Geometry: see drawing. Coordinates: mm, zero at the bounding-box minimum. A direction names the side the tool comes from. Give positions to 0.01 mm unless a question says otherwise; leave off trailing zeros. Order: outer loops, then holes, each group sorted by start corner. A loop starts at its lowest first (then second) coordinate and runs counter-clockwise, first axis right, second up. Notation, with made-up numbers: M -10.5,-2.75 L 39.5,-2.75 A17 cw 39.5,15.25 Z; hole C 32,14 d9. An arc over 180 degrees is marked long. Answer as a JSON object with one key per item and string values. Group by question number.
1. Material intervals for L1, parallel to X at y = 19, z = 31; L2, parallel to X at y = 49, z = 17; L3, parallel to Y at x = 16.25, z = 36, sorted ascending. Write a range as [from, to].
2. Section query B-B (x = 10). Output: boundary loops of the cut face in (y, z), plus the area to 3 significant figures.
3. Section query C-C (z = 25). Output: boundary loops of the cut face in (x, y), plus the area to 3 significant figures.
4. Section query D-D (y = 38). Output: boundary loops of the cut face in (x, z), plus the area to 3 significant figures.
5. Pin query (flat end, axial travel): P1, Ø4, axis at y = 28, z = 5.5, coming from the -X side; P2, Ø12, axis at y = 17.5, z = 23, coming from the +X side; P3, Ø2, axis at y = 40, z = 13, coming from the -X side. Return the tip coordinate at first contact, or that it passes through.
6. Section query A-A (y = 48). Output: boundary loops of the cut face in (x, z), plus the area to 3 significant figures.
7. Set-up query: the marked faces 1, 2 and 3. Return all of +Z, -Z, +X, -X, +Y, -Y with unobstructed straight access to the full face (end or side cutting, diameter ignored); none if empty.
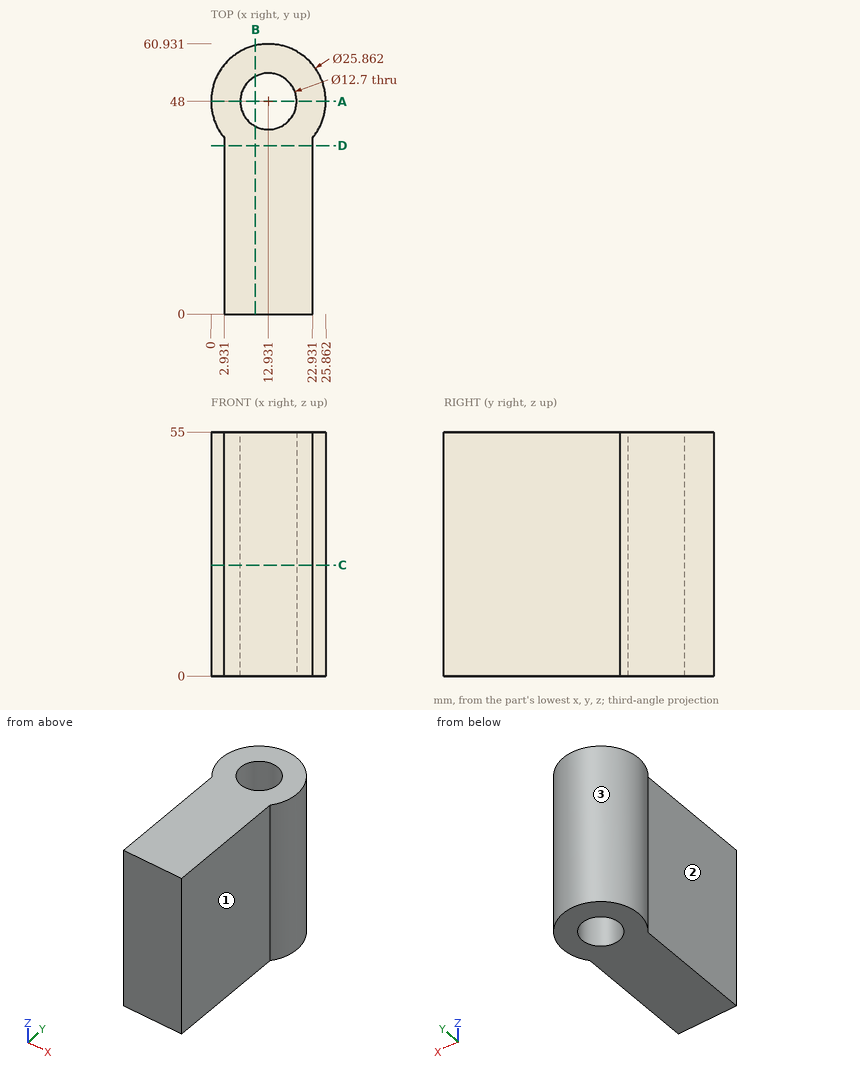
Answer sheet:
{
 "1": {"L1": "[2.93, 22.93]", "L2": "[0.04, 6.66], [19.2, 25.82]", "L3": "[0, 42.59], [53.41, 60.5]"},
 "2": {"outline": "M 0,0 L 42.37,0 L 42.37,55 L 0,55 Z; M 53.63,0 L 60.59,0 L 60.59,55 L 53.63,55 Z", "area": "2,710 mm^2"},
 "3": {"outline": "M 2.93,0 L 22.93,0 L 22.93,39.8 A12.93 ccw long 2.93,39.8 Z; hole C 12.93,48 d12.7", "area": "1,130 mm^2"},
 "4": {"outline": "M 2.93,0 L 22.93,0 L 22.93,55 L 2.93,55 Z", "area": "1,100 mm^2"},
 "5": {"P1": "x = 2.93", "P2": "x = 22.93", "P3": "x = 2.06"},
 "6": {"outline": "M 0,0 L 6.58,0 L 6.58,55 L 0,55 Z; M 19.28,0 L 25.86,0 L 25.86,55 L 19.28,55 Z", "area": "724 mm^2"},
 "7": {"face 1": "+Z, -Z, +X, -Y", "face 2": "+Z, -Z, -X, -Y", "face 3": "+Z, -Z"}
}
